```python
from build123d import *

# Parameters (mm, degrees)
BOSS_EXTRUDE1_DEPTH      = 40
BOSS_EXTRUDE1_DEPTH_BACK = 40
SKETCH1_R                = 25
SKETCH1_R_2              = 15
SKETCH2_R                = 10.000000000000002
BOSS_EXTRUDE2_DEPTH      = 13
SKETCH3_W                = 26.000000000000004
SKETCH3_H                = 40
BOSS_EXTRUDE3_DEPTH      = 3.645843
CUT_EXTRUDE1_DEPTH       = 102.36074190730847
BOSS_EXTRUDE4_DEPTH      = 10
SKETCH7_3_R              = 20
SKETCH7_3_R_2            = 12.500000000000002
BOSS_EXTRUDE5_DEPTH      = 20
SKETCH9_W                = 20
SKETCH9_H                = 40
BOSS_EXTRUDE6_DEPTH      = 2.087122
BOSS_EXTRUDE11_DEPTH     = 4.999999999999998


with BuildPart() as part:
    # Sketch1 → Boss-Extrude1 (new, two sides: drawn at the far end of the back side and taken through both)
    with BuildSketch(Plane(origin=(0, 0, 0), x_dir=(1, 0, 0), z_dir=(0, 1, 0)).offset(-BOSS_EXTRUDE1_DEPTH_BACK)):
        with Locations(Location((0, 0, 0), (0, 0, 270))):
            Circle(SKETCH1_R)
        with Locations(Location((0, 0, 0), (0, 0, 270))):
            Circle(SKETCH1_R_2, mode=Mode.SUBTRACT)
    extrude(amount=BOSS_EXTRUDE1_DEPTH + BOSS_EXTRUDE1_DEPTH_BACK)



with BuildPart() as body_2:
    # Sketch2 → Boss-Extrude2 (new, symmetric)
    with BuildSketch(Plane(origin=(0, 0, 0), x_dir=(0, 0, -1), z_dir=(1, 0, 0))):
        with BuildLine():
            Line((37, 40), (25, 40))
            Line((25, 40), (25, 0))
            Line((25, 0), (37, 0))
            ThreePointArc((37, 0), (57, 20), (37, 40))
        make_face()
        with Locations(Location((37, 20, 0), (0, 0, 180))):
            Circle(SKETCH2_R, mode=Mode.SUBTRACT)
    extrude(amount=BOSS_EXTRUDE2_DEPTH, both=True)


with BuildPart() as part_1:
    add(part.part)

    add(body_2.part)  # Boss-Extrude3 merges body 2
    # Sketch3 → Boss-Extrude3 (add)
    with BuildSketch(Plane.XY.offset(-25)):
        with Locations((0, 20)):
            Rectangle(SKETCH3_W, SKETCH3_H)
    extrude(amount=BOSS_EXTRUDE3_DEPTH)

    # Sketch4 → Cut-Extrude1 (cut, through all)
    with BuildSketch(Plane(origin=(0, 40, 0), x_dir=(1, 0, 0), z_dir=(0, 1, 0))):
        Polygon((-3.000000000000038, 151.757178913158), (2.9999999999999623, 151.75717891315796), (3.0000000000000093, -1.388e-14), (-2.999999999999991, -1.388e-14), align=None)
    extrude(amount=-CUT_EXTRUDE1_DEPTH, mode=Mode.SUBTRACT)



with BuildPart() as body_2_2:
    # Sketch7 → Boss-Extrude4 (new, symmetric)
    with BuildSketch(Plane(origin=(0, 0, 0), x_dir=(0, 0, -1), z_dir=(1, 0, 0))):
        with BuildLine():
            Line((-56.99999999999999, -40), (-25, -40))
            Line((-25, -40), (-25, 0))
            Line((-25, 0), (-56.99999999999999, 0))
            ThreePointArc((-56.99999999999999, 0), (-42.85786437626904, -5.857864376269051), (-36.99999999999999, -20))
            ThreePointArc((-36.99999999999999, -20.000000000000004), (-42.85786437626905, -34.14213562373095), (-57, -40))
        make_face()
    extrude(amount=BOSS_EXTRUDE4_DEPTH, both=True)

    # Sketch7<3> → Boss-Extrude5 (add, symmetric)
    with BuildSketch(Plane(origin=(0, 0, 0), x_dir=(0, 0, -1), z_dir=(1, 0, 0))):
        with Locations((-56.99999999999999, -20)):
            Circle(SKETCH7_3_R)
        with Locations((-56.99999999999999, -20)):
            Circle(SKETCH7_3_R_2, mode=Mode.SUBTRACT)
    extrude(amount=BOSS_EXTRUDE5_DEPTH, both=True)


with BuildPart() as part_2:
    add(part_1.part)

    add(body_2_2.part)  # Boss-Extrude6 merges body 2 2
    # Sketch9 → Boss-Extrude6 (add)
    with BuildSketch(Plane(origin=(0, 0, 25), x_dir=(-1, 0, 0), z_dir=(0, 0, -1))):
        with Locations((0, -20)):
            Rectangle(SKETCH9_W, SKETCH9_H)
    extrude(amount=BOSS_EXTRUDE6_DEPTH)

    # Sketch11 → Boss-Extrude11 (add, symmetric)
    with BuildSketch(Plane(origin=(0, 0, 0), x_dir=(0, 0, -1), z_dir=(1, 0, 0))):
        Polygon((-21.615437004072646, -2.0004940029139107), (-21.615437004072646, 38.49074239980155), (-25, 40), (-44.99999999999999, 0), (-44.99999999999999, -2.0004940029139107), align=None)
    extrude(amount=BOSS_EXTRUDE11_DEPTH, both=True)


solid = part_2.part
```
The listing builds one solid part. Answer for the finished solid, in the listing's coordinates (mm). A direction names the side the tool comes from. Coordinates: 2 decimals unless noted, no trailing zeros. Loops run counter-clockwise (first coordinate to the right, second up) from the corner with the lowest first, then second, coordinate; pieces in that order, holes last. Notation, with made-up numbers: (-6.75, 57) -> (40.25, 57) arc R20 cw to (40.25, 69) -> close; hole circle Ø2 at (76.25, 50.5). An arc over 180 degrees is marked (long way). Return JSON: item names as keys, results as strings. Group by question number.
(1) A cutting plane is placed at D-D on z = -28.5. Write down the section's boundary in (x, y), and give its area (3 significant figures).
(2) A cutting plane is placed at B-B on z = 0. Write down the section's boundary in (x, y).
(3) Determine the mould class of faces 5 (the flat face through (0, 20, 35)), 6 (the cylindrical face through (-0.28, -27.606, 66.92)), 7 (the flat face through (-20, -29, 66)) for opening direction Z: released by +Z, released by -Z, zero draft, split by the parting line, or undercut.
(4) Find the intervals of material crossed by probe 1 along Y at (x, z) = (7, -37); probe 2 along Z at (x, y) = (-11.5, -31.5); probe 3 along Z at (x, y) = (9.5, -28.5), in increasing order. Write a range as from..to.
(5) A cutting plane is placed at A-A on y = 20. Write down the section's boundary in (x, z), and give its area (3 significant figures).
(6) Which of the six approach directions +Z, -Z, +X, -X, +Y, -Y give full straight-line access (tool end or side, diameter ignored) to faces 1 (the flat face through (5, 16, 30)), 2 (the flat face through (-13, 19.7, -47.3)), 3 (the flat face through (13, 25, -47)), 4 (the flat face through (20, -29, 66))?
(7) Given pin 1 Ø16.5 at (y, z) = (28.5, 30) entering from -X; pin 2 Ø1 at (x, y) = (-11.5, 29) entering from +Z; pin 3 Ø8 at (x, z) = (8, -28.5) entering from -Y, each flat-ended and moving along its own axis, determine where each tip first touches the part or whether it passes through.
(8) A cutting plane is placed at C-C on x = -17.5. Write down the section's boundary in (y, z).
The answers:
{
 "1": {"outline": "(-13, 0) -> (-3, 0) -> (-3, 14.73) -> (-13, 14.73) -> close; (-13, 25.27) -> (-3, 25.27) -> (-3, 40) -> (-13, 40) -> close; (3, 0) -> (13, 0) -> (13, 14.73) -> (3, 14.73) -> close; (3, 25.27) -> (13, 25.27) -> (13, 40) -> (3, 40) -> close", "area": "589 mm^2"},
 "2": {"outline": "(-25, -40) -> (-15, -40) -> (-15, 40) -> (-25, 40) -> close; (15, -40) -> (25, -40) -> (25, 40) -> (15, 40) -> close"},
 "3": {"face 5": "released by +Z", "face 6": "undercut", "face 7": "zero draft"},
 "4": {"probe 1": "y = 0..10, 30..40", "probe 2": "z = -22.2..-9.63, 9.63..22.2, 40.64..52.1, 61.9..73.36", "probe 3": "z = -23.12..-11.61, 11.61..47.83, 66.17..75.1"},
 "5": {"outline": "(-13, -57) -> (-3, -57) -> (-3, -47) -> (-13, -47) -> close; (-13, -27) -> (-3, -27) -> (-3, -14.7) arc R15 cw (long way) to (3, -14.7) -> (3, -27) -> (13, -27) -> (13, -21.35) arc R25 ccw to (5, 24.49) -> (5, 35) -> (-5, 35) -> (-5, 24.49) arc R25 ccw to (-13, -21.35) -> close; (3, -57) -> (13, -57) -> (13, -47) -> (3, -47) -> close", "area": "1,570 mm^2"},
 "6": {"face 1": "+Z, +X, +Y", "face 2": "-Z, -X, +Y, -Y", "face 3": "-Z, +X, +Y, -Y", "face 4": "+Z, +X, +Y, -Y"},
 "7": {"pin 1": "stops at x = -12.33", "pin 2": "stops at z = 22.45", "pin 3": "stops at y = 0"},
 "8": {"outline": "(-40, -17.85) -> (40, -17.85) -> (40, 17.85) -> (-40, 17.85) -> close; circle Ø40 at (-20, 57); hole circle Ø25 at (-20, 57)"}
}
